Input: part model. Units: mm. Frame: model coordinates. A direction names the side the tool comes from. Round coordinates to 2 decimals unless told otherwise and drop trailing zeros. Write item = value, one per line.
```python
from build123d import *

# Parameters (mm, degrees)
SKETCH1_W                                       = 158.9
SKETCH1_H                                       = 114.98494382
BOSS_EXTRUDE1_DEPTH                             = 20
SKETCH2_R                                       = 44.45
CUT_EXTRUDE1_DEPTH                              = 5
SKETCH3_R                                       = 22.479
CUT_EXTRUDE2_DEPTH                              = 5.5
CSK_FOR_M6_FLAT_HEAD_MACHINE_SCREW1_D           = 6.6
CSK_FOR_M6_FLAT_HEAD_MACHINE_SCREW1_CSINK_D     = 12.6
CSK_FOR_M6_FLAT_HEAD_MACHINE_SCREW1_CSINK_ANGLE = 90
TAP_DRILL_FOR_M2X0_4_TAP1_D                     = 1.6
SKETCH18_W                                      = 20
SKETCH18_H                                      = 110
CUT_EXTRUDE3_DEPTH                              = 7.5
CSK_FOR_M6_FLAT_HEAD_MACHINE_SCREW2_D           = 6.6
CSK_FOR_M6_FLAT_HEAD_MACHINE_SCREW2_DEPTH       = 20
CSK_FOR_M6_FLAT_HEAD_MACHINE_SCREW2_CSINK_D     = 12.6
CSK_FOR_M6_FLAT_HEAD_MACHINE_SCREW2_CSINK_ANGLE = 90
CSK_FOR_M6_FLAT_HEAD_MACHINE_SCREW2_TIP         = 1.982840043


with BuildPart() as part:
    # Sketch1 → Boss-Extrude1 (new body)
    with BuildSketch(Plane(origin=(0, 0, 0), x_dir=(1, 0, 0), z_dir=(0, 1, 0))):
        Rectangle(SKETCH1_W, SKETCH1_H)
    extrude(amount=BOSS_EXTRUDE1_DEPTH)

    # Sketch2 → Cut-Extrude1 (cut)
    with BuildSketch(Plane.XZ):
        Circle(SKETCH2_R)
    extrude(amount=-CUT_EXTRUDE1_DEPTH, mode=Mode.SUBTRACT)

    # Sketch3 → Cut-Extrude2 (cut)
    with BuildSketch(Plane(origin=(0, 5, 0), x_dir=(-1, 0, 0), z_dir=(0, -1, 0))):
        Circle(SKETCH3_R)
    extrude(amount=-CUT_EXTRUDE2_DEPTH, mode=Mode.SUBTRACT)

    # CSK for M6 Flat Head Machine Screw1 (through all)
    with Locations(Plane(origin=(0, 20, 0), x_dir=(1, 0, 0), z_dir=(0, 1, 0))):
        with Locations((-17.5, 0), (-12.374368671, 12.374368671), (0, 17.5), (12.374368671, 12.374368671), (17.5, 0), (12.374368671, -12.374368671), (0, -17.5), (-12.374368671, -12.374368671)):
            CounterSinkHole(CSK_FOR_M6_FLAT_HEAD_MACHINE_SCREW1_D / 2, CSK_FOR_M6_FLAT_HEAD_MACHINE_SCREW1_CSINK_D / 2, counter_sink_angle=CSK_FOR_M6_FLAT_HEAD_MACHINE_SCREW1_CSINK_ANGLE)

    # Tap Drill for M2x0.4 Tap1 (through all)
    with Locations(Plane(origin=(0, 20, 0), x_dir=(1, 0, 0), z_dir=(0, 1, 0))):
        with Locations((-26.35, 0), (0, 26.35), (0, -26.35), (26.35, 0)):
            Hole(TAP_DRILL_FOR_M2X0_4_TAP1_D / 2)

    # Sketch18 → Cut-Extrude3 (cut)
    with BuildSketch(Plane(origin=(0, 20, 0), x_dir=(1, 0, 0), z_dir=(0, 1, 0))):
        with Locations((-54.45, 0)):
            Rectangle(SKETCH18_W, SKETCH18_H)
        with Locations((54.45, 0)):
            Rectangle(SKETCH18_W, SKETCH18_H)
    extrude(amount=-CUT_EXTRUDE3_DEPTH, mode=Mode.SUBTRACT)

    # CSK for M6 Flat Head Machine Screw2
    with Locations(Plane(origin=(0, 0, 0), x_dir=(-1, 0, 0), z_dir=(0, -1, 0))):
        with Locations((54.45, -36.666666667), (54.45, -18.333333333), (54.45, 0), (54.45, 18.333333333), (54.45, 36.666666667), (-54.45, 36.666666667), (-54.45, 18.333333333), (-54.45, 0), (-54.45, -18.333333333), (-54.45, -36.666666667)):
            CounterSinkHole(CSK_FOR_M6_FLAT_HEAD_MACHINE_SCREW2_D / 2, CSK_FOR_M6_FLAT_HEAD_MACHINE_SCREW2_CSINK_D / 2, depth=CSK_FOR_M6_FLAT_HEAD_MACHINE_SCREW2_DEPTH, counter_sink_angle=CSK_FOR_M6_FLAT_HEAD_MACHINE_SCREW2_CSINK_ANGLE)
            with Locations((0, 0, -(CSK_FOR_M6_FLAT_HEAD_MACHINE_SCREW2_DEPTH + CSK_FOR_M6_FLAT_HEAD_MACHINE_SCREW2_TIP / 2))):  # 118° drill point
                Cone(0, CSK_FOR_M6_FLAT_HEAD_MACHINE_SCREW2_D / 2, CSK_FOR_M6_FLAT_HEAD_MACHINE_SCREW2_TIP, mode=Mode.SUBTRACT)


solid = part.part
```
1) Access query for faces 1 (the face through (64.45, 16, 1)), 2 (the face through (0, 10.5, 0)), 3 (the face through (-57.1, 7.8, 20.3)). Directions: +Z, -Z, +X, -X, +Y, -Y. A direction counts if a zero-diameter tool reaches every point of the face in a straight line with its end or side. Return the directions, or none.
Solutions:
face_1 = +Y
face_2 = -Y
face_3 = +Y, -Y
2) Line query: L1, parallel to Z at x = 0, y = 8.35; L2, parallel to X at y = 4.25, z = 0.5; L3, parallel to X at y = 16.5, z = -26.35. Output: solid intervals per line, ascending. Write a range as from..to.
Solutions:
L1 = -57.49..-27.15, -25.55..-22.48, 22.48..25.55, 27.15..57.49
L2 = -79.45..-57.71, -51.19..-44.45, 44.45..51.19, 57.71..79.45
L3 = -79.45..-64.45, -44.45..-0.8, 0.8..44.45, 64.45..79.45
3) Draft query along Z for faces 4 (the face through (-1, 10, 57.492)), 5 (the face through (53.7, 2.85, -33.3)). Return one class per face: +Z half, -Z half, draft (parallel to the pull), parting line (faces both ways), or undercut.
Solutions:
face_4 = +Z half
face_5 = undercut
4) First-contact query: P1, Ø8.5, axis at x = -54.45, z = -36.67, coming from the +Y side; P2, Ø10.5, axis at x = 54.45, z = 0, coming from the -Y side; P3, Ø1.8, axis at x = -26.35, z = 0, coming from the -Y side; P4, Ø12, axis at x = 62, z = 27, coming from the -Y side. Flat tips, straight axial feed; report the tip coordinate or a pass-through.
Solutions:
P1 = 12.5
P2 = 1.05
P3 = 5
P4 = 0
5) Cut plane A-A (y = 7.75). Count the separate pieces of the cut face and the enclosed holes in it, and give its area (3 significant figures).
Solutions:
separate_pieces = 1
enclosed_holes = 15
area = 16,300 mm^2
